The model under review builds one solid part; all positions refer to its coordinate system, in mm. A direction names the side the tool comes from. Give positions to 0.01 mm unless a question says otherwise; leave off trailing zeros. Loops run counter-clockwise (first coordinate to the right, second up) from the corner with the lowest first, then second, coordinate; pieces in that order, holes last. Notation, with made-up numbers: M 59,70.5 L 87,70.5 A26 ccw 87,88.5 Z; hole C -7,87.5 d10. An arc over 180 degrees is marked long. Return JSON: item names as keys, results as strings.
```python
from build123d import *

# Parameters (mm, degrees)
SKETCH1_W           = 37
SKETCH1_H           = 17
BOSS_EXTRUDE1_DEPTH = 11
SHELL1_T            = -1
SKETCH2_W           = 10
SKETCH2_H           = 3.5
CUT_EXTRUDE1_DEPTH  = 11
SKETCH3_R           = 1.5
SKETCH3_W           = 8
SKETCH3_H           = 8
CUT_EXTRUDE2_DEPTH  = 2


with BuildPart() as part:
    # Sketch1 → Boss-Extrude1 (new body)
    with BuildSketch(Plane(origin=(0, 0, 0), x_dir=(1, 0, 0), z_dir=(0, 1, 0))):
        Rectangle(SKETCH1_W, SKETCH1_H)
    extrude(amount=BOSS_EXTRUDE1_DEPTH)

    # Shell1
    shell1_openings = [part.faces().sort_by_distance(p)[0] for p in [
        (18.5, 5.5, 0),
    ]]
    offset(amount=SHELL1_T, openings=shell1_openings, kind=Kind.INTERSECTION)

    # Sketch2 → Cut-Extrude1 (cut)
    with BuildSketch(Plane.ZY.offset(18.5)):
        with Locations((0, 7.75)):
            Rectangle(SKETCH2_W, SKETCH2_H)
    extrude(amount=-CUT_EXTRUDE1_DEPTH, mode=Mode.SUBTRACT)

    # Sketch3 → Cut-Extrude2 (cut)
    with BuildSketch(Plane(origin=(0, 11, 0), x_dir=(1, 0, 0), z_dir=(0, 1, 0))):
        with Locations(Location((-11, 0, 0), (0, 0, 270))):
            Circle(SKETCH3_R)
        with Locations((-2, -3.5)):
            Rectangle(SKETCH3_W, SKETCH3_H)
    extrude(amount=-CUT_EXTRUDE2_DEPTH, mode=Mode.SUBTRACT)


solid = part.part
```
1) Consider section C-C on y = 8.5. Write out the cut boundary in (x, z).
From the geometry:
{"outline": "M -18.5,-8.5 L 18.5,-8.5 L 18.5,-7.5 L -17.5,-7.5 L -17.5,-5 L -18.5,-5 Z; M -18.5,5 L -17.5,5 L -17.5,7.5 L 18.5,7.5 L 18.5,8.5 L -18.5,8.5 Z"}
2) Wall thickness on L1, parallel to X at y = 10.7, z = 0; L2, parallel to X at y = 10.25, z = 4; L3, parallel to Z at x = 16, y = 4.25: over which ranges is each line inside the solid? List them lowest first. Write a range as from..to.
From the geometry:
{"L1": "-18.5..-12.5, -9.5..-6, 2..18.5", "L2": "-18.5..-6, 2..18.5", "L3": "-8.5..-7.5, 7.5..8.5"}
3) The part is to be moulded in two halves that separate along Z. For faces 4 (the face through (0, 5, 8.5)), 5 (the face through (0, 0, 0)), 6 (the face through (-18, 6, 0)), say which applies: released by +Z, released by -Z, zero draft, split by the parting line, or undercut.
From the geometry:
{"face 4": "released by +Z", "face 5": "zero draft", "face 6": "undercut"}
4) Tool access review of faces 1 (the face through (-18, 8, 5)), 2 (the face through (-12.464, 10.507, -0.325)), 3 (the face through (0, 10, -2)): name each direction out of +Z, -Z, +X, -X, +Y, -Y from which nothing blocks a thin tool from reaching the whole face with its end or side.
From the geometry:
{"face 1": "+X, -X", "face 2": "+Y", "face 3": "+X"}
5) Consider section B-B on z = 3. Write out the cut boundary in (x, y), then the cut area to 3 significant figures.
From the geometry:
{"outline": "M -18.5,0 L 18.5,0 L 18.5,1 L -17.5,1 L -17.5,6 L -18.5,6 Z; M -18.5,9.5 L -17.5,9.5 L -17.5,10 L -6,10 L -6,11 L -18.5,11 Z; M 2,10 L 18.5,10 L 18.5,11 L 2,11 Z", "area": "71.5 mm²"}
6) Consider section D-D on x = 16.5. Write out the cut boundary in (y, z), then the cut area to 3 significant figures.
From the geometry:
{"outline": "M 0,-8.5 L 11,-8.5 L 11,8.5 L 0,8.5 Z; hole M 1,-7.5 L 10,-7.5 L 10,7.5 L 1,7.5 Z", "area": "52.0 mm²"}
7) Consider section A-A on z = 6.5. Write out the cut boundary in (x, y), then the cut area to 3 significant figures.
From the geometry:
{"outline": "M -18.5,0 L 18.5,0 L 18.5,1 L -17.5,1 L -17.5,10 L -6,10 L -6,11 L -18.5,11 Z; M 2,10 L 18.5,10 L 18.5,11 L 2,11 Z", "area": "75.0 mm²"}
